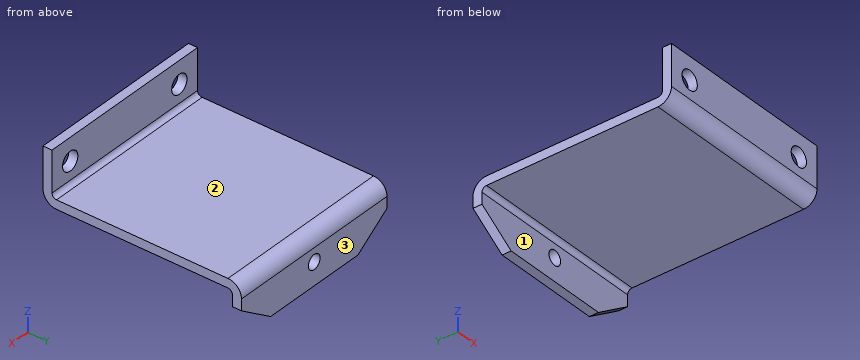
from build123d import *

# Parameters (mm, degrees)
SKETCH_2_W            = 40
SKETCH_2_H            = 10
SKETCH_2_R            = 2.1
EXTRUDE_1_DEPTH       = 2
SKETCH_3_W            = 40
SKETCH_3_H            = 44
EXTRUDE_2_DEPTH       = 2
SKETCH_4_W            = 40
SKETCH_4_H            = 11
SKETCH_4_R            = 1.6
EXTRUDE_3_DEPTH       = 2
CUT_EXTRUDE_1_DEPTH   = 51.911688245
SHEET_START           = -20
SHEET_METAL_1_DEPTH   = 40
SHEET_METAL_1_2_DEPTH = 40


# Read off the part's stored shape, not the designer's step: 转换实体1
with BuildPart() as part:
    # Sketch 2 → 凸台-拉伸1 (new body)
    with BuildSketch(Plane(origin=(0, 0, 0), x_dir=(1, 0, 0), z_dir=(0, 1, 0))):
        Rectangle(SKETCH_2_W, SKETCH_2_H)
        with Locations(Location((-15, 0, 0), (0, 0, 270))):
            Circle(SKETCH_2_R, mode=Mode.SUBTRACT)
        with Locations(Location((15, 0, 0), (0, 0, 90))):
            Circle(SKETCH_2_R, mode=Mode.SUBTRACT)
    extrude(amount=EXTRUDE_1_DEPTH)

    # 草图3 → 凸台-拉伸2 (add)
    with BuildSketch(Plane(origin=(0, 0, -5), x_dir=(-1, 0, 0), z_dir=(0, 0, -1))):
        with Locations((0, 22)):
            Rectangle(SKETCH_3_W, SKETCH_3_H)
    extrude(amount=EXTRUDE_2_DEPTH)

    # 草图4 → 凸台-拉伸3 (add)
    with BuildSketch(Plane(origin=(0, 44, 0), x_dir=(1, 0, 0), z_dir=(0, 1, 0))):
        with Locations((0, 10.5)):
            Rectangle(SKETCH_4_W, SKETCH_4_H)
        with Locations(Location((0, 11, 0), (0, 0, 270))):
            Circle(SKETCH_4_R, mode=Mode.SUBTRACT)
    extrude(amount=-EXTRUDE_3_DEPTH)

    # 草图5 → 切除-拉伸1 (cut, through all)
    with BuildSketch(Plane(origin=(0, 44, 0), x_dir=(1, 0, 0), z_dir=(0, 1, 0))):
        Polygon((-20, 16), (-20, 10.5), (-12, 16), align=None)
        Polygon((20, 10.5), (12, 16), (20, 16), align=None)
    extrude(amount=-CUT_EXTRUDE_1_DEPTH, mode=Mode.SUBTRACT)

    # Sheet Metal 1 outline → Sheet Metal 1 (cut)
    with BuildSketch(Plane.YZ.offset(SHEET_START)):
        with BuildLine():
            Line((44, -5), (41, -5))
            ThreePointArc((41, -5), (43.121320344, -5.878679656), (44, -8))
            Line((44, -8), (44, -5))
        make_face()
        with BuildLine():
            ThreePointArc((3, -7), (0.878679656, -6.121320344), (0, -4))
            Line((0, -4), (0, -7))
            Line((0, -7), (3, -7))
        make_face()
    extrude(amount=SHEET_METAL_1_DEPTH, mode=Mode.SUBTRACT)

    # Sheet Metal 1 2 outline → Sheet Metal 1 2 (add)
    with BuildSketch(Plane.YZ.offset(SHEET_START)):
        with BuildLine():
            ThreePointArc((3, -5), (2.292893219, -4.707106781), (2, -4))
            Line((2, -4), (2, -5))
            Line((2, -5), (3, -5))
        make_face()
        with BuildLine():
            Line((42, -7), (41, -7))
            ThreePointArc((41, -7), (41.707106781, -7.292893219), (42, -8))
            Line((42, -8), (42, -7))
        make_face()
    extrude(amount=SHEET_METAL_1_2_DEPTH)


solid = part.part
CAD build for the part. Positions are in the model's coordinates, mm. Face numbers are marked on the shaded views. A direction names the side the tool comes from. Give positions to 0.01 mm unless a question says otherwise; leave off trailing zeros. Loops run counter-clockwise (first coordinate to the right, second up) from the corner with the lowest first, then second, coordinate; pieces in that order, holes last. Notation, with made-up numbers: M -21,15.5 L 16,15.5 A5 ccw 16,24.5 Z; hole C -22.5,-22 d9. An arc over 180 degrees is marked long. Answer in a Markdown table with one row per item. Add a question column.
Item 1: Probe probe 1 along X at (y, z) = (1.35, 0); probe 2 along Z at (x, y) = (-5, 41); probe 3 along Y at (x, z) = (-14.5, -12). List the from-to ranges inside material, lowest first.
Item 2: Band-saw the part on C-C on z = -3. Give the cut face in (x, y).
Item 3: Band-saw the part on A-A on x = 0. Give the cut face in (y, z), then the cut area to 3 significant figures.
Item 4: Band-saw the part on D-D on y = 19. Give the cut face in (x, z), then the cut area to 3 significant figures.
Item 5: Tool access for the marked faces 1, 2 and 3: list every direction of +Z, -Z, +X, -X, +Y, -Y with a clear straight run to the whole face (end or side of a thin tool).
Item 6: Band-saw the part on B-B on x = -9. Give the cut face in (y, z).
Item 7: Drop flat-ended pins along their axis: P1, Ø6, axis at y = 32.5, z = -11, coming from the -X side; P2, Ø19, axis at x = -1.5, y = 16.5, coming from the -Z side; P3, Ø2.5, axis at x = -2, z = 1.5, coming from the +Y side; P4, Ø8, axis at x = 7.5, z = -10.5, coming from the -Y side. Give the stop position or say it passes through.
Reply:
| question | item | result |
|---|---|---|
| 1 | probe 1 | x = -20 to -17.1, -12.9 to 12.9, 17.1 to 20 |
| 1 | probe 2 | z = -7 to -5 |
| 1 | probe 3 | y = 42 to 44 |
| 2 | outline | M -20,0 L 20,0 L 20,2 L -20,2 Z |
| 3 | outline | M 0,-4 A3 ccw 3,-7 L 41,-7 A1 cw 42,-8 L 42,-9.4 L 44,-9.4 L 44,-8 A3 ccw 41,-5 L 3,-5 A1 cw 2,-4 L 2,5 L 0,5 Z; M 42,-16 L 44,-16 L 44,-12.6 L 42,-12.6 Z |
| 3 | area | 116 mm^2 |
| 4 | outline | M -20,-7 L 20,-7 L 20,-5 L -20,-5 Z |
| 4 | area | 80.0 mm^2 |
| 5 | face 1 | -Z, +X, -X, -Y |
| 5 | face 2 | +Z, +X, -X, +Y |
| 5 | face 3 | +Z, -Z, +X, -X, +Y |
| 6 | outline | M 0,-4 A3 ccw 3,-7 L 41,-7 A1 cw 42,-8 L 42,-16 L 44,-16 L 44,-8 A3 ccw 41,-5 L 3,-5 A1 cw 2,-4 L 2,5 L 0,5 Z |
| 7 | P1 | passes through |
| 7 | P2 | stops at z = -7 |
| 7 | P3 | stops at y = 2 |
| 7 | P4 | stops at y = 1.34 |
